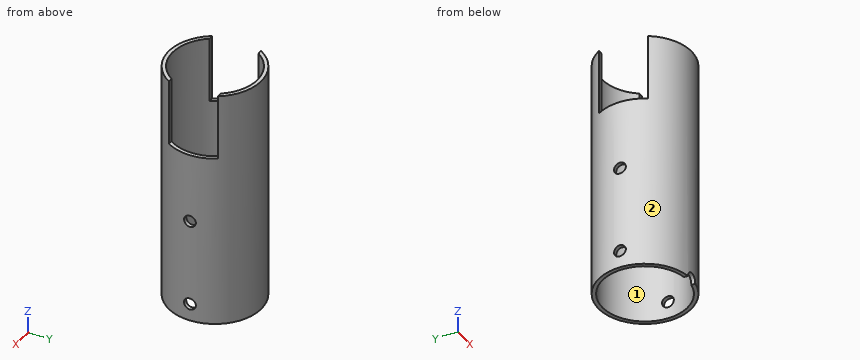
from build123d import *

# Parameters (mm, degrees)
SKETCH_1_R               = 24
SKETCH_1_R_2             = 22
EXTRUDE_1_DEPTH          = 124
SKETCH_2_R               = 3.5
CUT_EXTRUDE_1_DEPTH      = 100
CUT_EXTRUDE_2_DEPTH      = 129.561269574
CUT_EXTRUDE_2_DEPTH_BACK = 129.561269574
SKETCH_3_W               = 68
SKETCH_3_H               = 25
CUT_EXTRUDE_3_DEPTH      = 129.561269574
CUT_EXTRUDE_3_DEPTH_BACK = 129.561269574
SKETCH_4_R               = 3


with BuildPart() as part:
    # 草图1 → 凸台-拉伸1 (new body)
    with BuildSketch(Plane.XY):
        Circle(SKETCH_1_R)
        Circle(SKETCH_1_R_2, mode=Mode.SUBTRACT)
    extrude(amount=EXTRUDE_1_DEPTH)

    # 草图2 → 切除-拉伸1 (cut)
    with BuildSketch(Plane(origin=(0, 0, 0), x_dir=(1, 0, 0), z_dir=(0, 1, 0))):
        Circle(SKETCH_2_R)
    extrude(amount=-CUT_EXTRUDE_1_DEPTH, mode=Mode.SUBTRACT)

    # 草图3 → 切除-拉伸2 (cut, two sides: drawn at the far end of the back side and taken through both)
    with BuildSketch(Plane(origin=(0, 0, 0), x_dir=(0, 0, -1), z_dir=(1, 0, 0)).offset(-CUT_EXTRUDE_2_DEPTH_BACK)):
        with Locations((-124, 0)):
            Rectangle(SKETCH_3_W, SKETCH_3_H)
    extrude(amount=CUT_EXTRUDE_2_DEPTH + CUT_EXTRUDE_2_DEPTH_BACK, mode=Mode.SUBTRACT)

    # 草图4 → 切除-拉伸3 (cut, two sides: drawn at the far end of the back side and taken through both)
    with BuildSketch(Plane(origin=(0, 0, 0), x_dir=(0, 0, -1), z_dir=(1, 0, 0)).offset(-CUT_EXTRUDE_3_DEPTH_BACK)):
        with Locations((-9, 0)):
            Circle(SKETCH_4_R)
        with Locations((-54, 0)):
            Circle(SKETCH_4_R)
    extrude(amount=CUT_EXTRUDE_3_DEPTH + CUT_EXTRUDE_3_DEPTH_BACK, mode=Mode.SUBTRACT)


solid = part.part
Can you work these out from the model? Positions are in its coordinate system, mm. Face numbers are marked on the shaded views. Give positions to 0.01 mm unless a question says otherwise; leave off trailing zeros. Order: outer loops, then holes, each group sorted by start corner. A loop starts at its lowest first (then second) coordinate and runs counter-clockwise, first axis right, second up. Notation, with made-up numbers: M 23,22.25 L 52,22.25 A28 ccw 52,46.25 Z; hole C 34.25,25.5 d8. An arc over 180 degrees is marked long. Use one line per item in the form item = value. Start each with the question number.
Item 1: If we section it at A-A (x = 0): Write out the boundary of the cut face in (y, z).
Item 2: We'd pull the mould along X, two halves only. Please class the marked faces 1 and 2: +X half, -X half, draft (parallel to the pull), parting line (faces both ways), or undercut.
Item 3: If we section it at D-D (z = 33): Write out the boundary of the cut face in (x, y), then the cut area to 3 significant figures.
Item 4: If I drill on line 1 along Z through (x, y) = (-23, 0); line 2 along X through (y, z) = (0, 41); line 3 along Y through (x, z) = (12.5, 76), over which ranges is the centre line in solid material (lowest first)?
Item 5: Will these pins go through, and if not, where does the flat tip stop? pin 1 Ø2.5 at (x, z) = (18.5, 108.5) entering from +Y; pin 2 Ø1.8 at (x, y) = (22, 1.5) entering from +Z; pin 3 Ø0.7 at (x, z) = (-19, 99) entering from -Y.
Item 6: If we section it at C-C (z = 9): Write out the boundary of the cut face in (x, y), then the cut area to 3 significant figures.
Item 7: If we section it at B-B (y = 0): Write out the boundary of the cut face in (x, z), then the cut area to 3 significant figures.
Outcome:
q1.outline = M -24,3.5 L -22,3.5 L -22,124 L -24,124 Z; M 22,0 L 24,0 L 24,124 L 22,124 Z
q2.face_1 = undercut
q2.face_2 = parting line
q3.outline = C 0,0 d48; hole C 0,0 d44
q3.area = 289 mm2
q4.line_1 = 0 to 6, 12 to 51, 57 to 90
q4.line_2 = -24 to -22, 22 to 24
q4.line_3 = -20.49 to -18.1, 18.1 to 20.49
q5.pin_1 = 16.69
q5.pin_2 = 90
q5.pin_3 = -15.11
q6.outline = M -23.81,-3 A24 ccw 23.81,-3 L 21.79,-3 A22 cw -21.79,-3 Z; M -23.81,3 L -21.79,3 A22 cw 21.79,3 L 23.81,3 A24 ccw Z
q6.area = 265 mm2
q7.outline = M -24,0 L -22,0 L -22,6 L -24,6 Z; M -24,12 L -22,12 L -22,51 L -24,51 Z; M -24,57 L -22,57 L -22,90 L -24,90 Z; M 22,0 L 24,0 L 24,6 L 22,6 Z; M 22,12 L 24,12 L 24,51 L 22,51 Z; M 22,57 L 24,57 L 24,90 L 22,90 Z
q7.area = 312 mm2
